Part model, mm, in its own coordinate system. A direction names the side the tool comes from. Give positions to 0.01 mm unless a question says otherwise; leave off trailing zeros. Order: outer loops, then holes, each group sorted by start corner. A loop starts at its lowest first (then second) coordinate and runs counter-clockwise, first axis right, second up. Notation, with made-up numbers: M 31.25,7.25 L 72.25,7.25 A4 ccw 72.25,11.25 Z; hole C 57.5,11 d11. An arc over 180 degrees is marked long. Return JSON: item names as keys, results as strings.
from build123d import *

# Parameters (mm, degrees)
F0_R           = 15
F1_DEPTH       = 2
F2_R           = 23.5
F3_DEPTH       = 8
F4_R           = 12
F5_DEPTH       = 3
F6_R           = 7.5
F7_DEPTH       = 7.001
F9_D           = 4.4
F9_CBORE_D     = 8
F9_CBORE_DEPTH = 4


with BuildPart() as f1:
    # F0 (on Top) → F1 (new body)
    with BuildSketch(Plane.XY):
        Circle(F0_R)
    extrude(amount=-F1_DEPTH)

    # F2 (on Top) → F3 (join)
    with BuildSketch(Plane.XY):
        Circle(F2_R)
    extrude(amount=F3_DEPTH)

    # F4 (on face) → F5 (cut)
    with BuildSketch(Plane.XY.offset(8)):
        Circle(F4_R)
    extrude(amount=-F5_DEPTH, mode=Mode.SUBTRACT)

    # F6 (on face) → F7 (cut, through all)
    with BuildSketch(Plane.XY.offset(5)):
        Circle(F6_R)
    extrude(amount=-F7_DEPTH, mode=Mode.SUBTRACT)

    # F9 (through all)
    with Locations(Plane.XY.offset(8)):
        with Locations((0, 18.5), (-18.5, 0), (0, -18.5), (18.5, 0)):
            CounterBoreHole(F9_D / 2, F9_CBORE_D / 2, F9_CBORE_DEPTH)


solid = f1.part
Q1. Band-saw the part on C-C (y = -5.5). Give the cut face in (x, z), then the cut area to 3 significant figures.
Established:
{"outline": "M -22.85,0 L -13.96,0 L -13.96,-2 L -5.1,-2 L -5.1,5 L -10.67,5 L -10.67,8 L -22.85,8 Z; M 5.1,-2 L 13.96,-2 L 13.96,0 L 22.85,0 L 22.85,8 L 10.67,8 L 10.67,5 L 5.1,5 Z", "area": "286 mm²"}
Q2. Band-saw the part on A-A (x = 0). Give the number of separate pieces and of enclosed holes in the cut face, then the cut area to 3 significant figures.
Established:
{"separate pieces": "4", "enclosed holes": "0", "area": "160 mm²"}
Q3. Band-saw the part on D-D (z = 6.5). Give the cut face in (x, y), then the cut area to 3 significant figures.
Established:
{"outline": "C 0,0 d47; hole C -18.5,0 d8; hole C 0,0 d24; hole C 0,-18.5 d8; hole C 0,18.5 d8; hole C 18.5,0 d8", "area": "1,080 mm²"}
Q4. Pin check, flat tips, straight feed: pin 1 (7 mm diameter, centred on x = 0, y = 18.5, fed in from +Z); pin 2 (1.5 mm diameter, centred on x = -4, z = 2, fed in from -Y); pin 3 (5.5 mm diameter, centred on x = 0, y = -18.5, fed in from -Z); pin 4 (3.5 mm diameter, centred on x = -18.5, y = 0, fed in from -Z). Stop position of each tip, or through.
Established:
{"pin 1": "stops at z = 4", "pin 2": "stops at y = -23.27", "pin 3": "stops at z = 0", "pin 4": "passes through"}
Q5. Two-plate mould, pull along X, no slides. Class faces 1 (the cylindrical face through (-0.521, -14.534, 6.028)), 2 (the cylindrical face through (22.4, 7.1, 3.9)), 3 (the flat face through (-4, 7, -2)): +X half, -X half, draft (parallel to the pull), parting line (faces both ways), or undercut.
Established:
{"face 1": "undercut", "face 2": "parting line", "face 3": "draft"}
Q6. 3-axis set-ups, long thin cutter, end or side, ignore diameter. For faces 4 (the cylindrical face through (15.3, -2.4, 6)), 5 (the cylindrical face through (16.468, -0.843, 1.972)), 6 (the flat face through (-11, 11, 0)): which of +Z, -Z, +X, -X, +Y, -Y reach the whole face in a straight line?
Established:
{"face 4": "+Z", "face 5": "+Z, -Z", "face 6": "-Z"}
Q7. Probe line 1 along Z through (x, y) = (-20, 9); line 2 along Z through (x, y) = (-8, -5); line 3 along X through (y, z) = (-4.5, 6.5). List the from-to ranges inside material, lowest first.
Established:
{"line 1": "z = 0 to 8", "line 2": "z = -2 to 5", "line 3": "x = -23.07 to -11.12, 11.12 to 23.07"}
